CAD build for the part. Positions are in the model's coordinates, mm. A direction names the side the tool comes from. Round coordinates to 2 decimals unless told otherwise and drop trailing zeros. Loops run counter-clockwise (first coordinate to the right, second up) from the corner with the lowest first, then second, coordinate; pieces in that order, holes last. Notation, with made-up numbers: M 34,11.25 L 44,11.25 A27 cw 44,31.25 Z; hole C 83,-9 d6. An arc over 180 degrees is marked long. Use one line per item in the form item = value.
from build123d import *

# Parameters (mm, degrees)
D_GAGEMENT_M51_D             = 5.5
R_P_TITION_CIRCULAIRE1_COUNT = 2
R_P_TITION_CIRCULAIRE1_ANGLE = 90
ESQUISSE5_W                  = 3
ESQUISSE5_H                  = 15
ENL_V_MAT_EXTRU_1_DEPTH      = 10
R_P_TITION_CIRCULAIRE2_COUNT = 4


with BuildPart() as part:
    # Esquisse1 → Révolution1 (revolve)
    with BuildSketch(Plane.XY):
        Polygon((0, 37.65), (10, 37.65), (10, 39), (20, 39), (20, 42), (0, 42), align=None)
    revolve(axis=Axis((0, 0, 0), (1, 0, 0)))

    # Dégagement M51 (through all)
    with Locations(Plane(origin=(16, 42, 0), x_dir=(0, 0, 1), z_dir=(0, 1, 0))):
        with Locations((0, 0)):
            d_gagement_m51 = Hole(D_GAGEMENT_M51_D / 2)

    # Répétition circulaire1: Dégagement M51 ×2 about axis
    r_p_tition_circulaire1_axis = Axis((20, 0, 0), (-1, 0, 0))
    for i in range(1, R_P_TITION_CIRCULAIRE1_COUNT):
        add(d_gagement_m51.rotate(r_p_tition_circulaire1_axis, i * R_P_TITION_CIRCULAIRE1_ANGLE / (R_P_TITION_CIRCULAIRE1_COUNT - 1)), mode=Mode.SUBTRACT)

    # Esquisse5 → Enlèv. mat.-Extru.1 (cut)
    with BuildSketch(Plane.ZY):
        with Locations((0, 47.5)):
            Rectangle(ESQUISSE5_W, ESQUISSE5_H)
    enl_v_mat_extru_1 = extrude(amount=-ENL_V_MAT_EXTRU_1_DEPTH, mode=Mode.SUBTRACT)

    # Répétition circulaire2: Enlèv. mat.-Extru.1 ×4 about axis
    r_p_tition_circulaire2_axis = Axis((0, 0, 0), (1, 0, 0))
    for i in range(1, R_P_TITION_CIRCULAIRE2_COUNT):
        add(enl_v_mat_extru_1.rotate(r_p_tition_circulaire2_axis, i * 360 / R_P_TITION_CIRCULAIRE2_COUNT), mode=Mode.SUBTRACT)


solid = part.part
1. Cut at C-C on x = 6.25. Write the cut outline in (y, z).
Completed:
outline = M -41.97,-1.5 A42 ccw -1.5,-41.97 L -1.5,-40 L 1.5,-40 L 1.5,-41.97 A42 ccw 41.97,-1.5 L 40,-1.5 L 40,1.5 L 41.97,1.5 A42 ccw 1.5,41.97 L 1.5,40 L -1.5,40 L -1.5,41.97 A42 ccw -41.97,1.5 L -40,1.5 L -40,-1.5 Z; hole C 0,0 d75.3
2. Cut at A-A on y = 0. Write the cut outline in (x, z).
Completed:
outline = M 0,-40 L 10,-40 L 10,-42 L 13.25,-42 L 13.25,-39 L 10,-39 L 10,-37.65 L 0,-37.65 Z; M 0,37.65 L 10,37.65 L 10,39 L 13.25,39 L 13.25,42 L 10,42 L 10,40 L 0,40 Z; M 18.75,-42 L 20,-42 L 20,-39 L 18.75,-39 Z; M 18.75,39 L 20,39 L 20,42 L 18.75,42 Z
3. Tool access for faces 3 (the face through (5, -1.5, -41)), 4 (the face through (10, 0, 41)), 5 (the face through (5, -40, 0)): list every direction of +Z, -Z, +X, -X, +Y, -Y with a clear straight run to the whole face (end or side of a thin tool).
Completed:
face_3 = -Z, -X
face_4 = +Z, -X
face_5 = -X, -Y
4. Drop flat-ended pins along their axis: P1, Ø0.6, axis at y = 0, z = 41, coming from the -X side; P2, Ø12, axis at x = 5.5, z = -28, coming from the +Y side; P3, Ø5, axis at x = 5, z = -31.5, coming from the +Y side. Give the stop position or say it passes through.
Completed:
P1 = 10
P2 = 35.78
P3 = 30.38
5. Cut at D-D on z = 20. Write the cut outline in (x, y).
Completed:
outline = M 0,-36.93 L 20,-36.93 L 20,-33.48 L 10,-33.48 L 10,-31.9 L 0,-31.9 Z; M 0,31.9 L 10,31.9 L 10,33.48 L 20,33.48 L 20,36.93 L 0,36.93 Z
6. Pull direction Z, two halves, no side cores. Call faces 1 (the face through (5, 1.5, -41)), 2 (the face through (18.727, -40.473, 0.358)): +Z half, -Z half, draft (parallel to the pull), parting line (faces both ways), or undercut.
Completed:
face_1 = draft
face_2 = undercut
7. Probe line 1 along Z through (x, y) = (13, 0); line 2 along Z through (x, y) = (12.5, 6); line 3 along Y through (x, z) = (5.5, -3). List the from-to ranges inside material, lowest first. Write a range as from..to.
Completed:
line_1 = -42..-39, 39..42
line_2 = -41.57..-38.54, 38.54..41.57
line_3 = -41.89..-37.53, 37.53..41.89
